Autodesk Inventor part; units mm, degrees
ref_plane "YZ Plane" through (0, 0, 0) normal (1, 0, 0) x (0, 1, 0)
ref_plane "XZ Plane" through (0, 0, 0) normal (0, 1, 0) x (-1, 0, 0)
ref_plane "XY Plane" through (0, 0, 0) normal (0, 0, 1) x (1, 0, 0)
sketch "Sketch1" plane through (0, 0, 0) normal (0, 1, 0) x (-1, 0, 0)
  line L0 (-12.7, -12.7) -> (12.7, -12.7)
  line L1 (12.7, -12.7) -> (12.7, 12.7)
  line L2 (12.7, 12.7) -> (-12.7, 12.7)
  line L3 (-12.7, 12.7) -> (-12.7, -12.7)
  line L4 (-12.7, -12.7) -> (12.7, 12.7) construction
  line L5 (12.7, -12.7) -> (-12.7, 12.7) construction
  line L6 (9.525, 9.525) -> (9.525, -9.525)
  line L7 (9.525, -9.525) -> (-9.525, -9.525)
  line L8 (-9.525, -9.525) -> (-9.525, 9.525)
  line L9 (-9.525, 9.525) -> (9.525, 9.525)
  point P0 (0, 0)
  dimension "d0" = 25.4
  dimension "d1" = 25.4
  dimension "d2" = 3.175
extrude "Extrusion1" add sketch "Sketch1" along normal blind 514.35
sketch "Sketch2" plane through (12.7, 0, 12.7) normal (1, 0, 0) x (0, 0, -1)
  line L0 (25.4, 514.35) -> (0, 514.35)
  line L1 (0, 514.35) -> (25.4, 488.95)
  line L2 (25.4, 0) -> (25.4, 514.35)
  circle A0 centre (12.7, 482.6) radius 3.2512
  line L3 (0, 514.35) -> (25.4, 514.35)
  circle A1 centre (12.7, 463.55) radius 3.2512
  circle A2 centre (12.7, 501.65) radius 3.2512
  point P0 (12.7, 0)
  point P1 (12.7, 514.35)
  point P2 (12.7, 514.35)
  point P3 (14.9989, 499.3511)
  point P4 (10.4011, 503.9489)
  dimension "d5" = 25.4
  dimension "d6" = 6.5024
  dimension "d7" = 31.75
  dimension "d8" = 19.05
extrude "Extrusion2" cut sketch "Sketch2" against normal blind 522.224
sketch "Sketch3" plane through (0, 0, 0) normal (0, -1, 0) x (1, 0, 0)
  line L0 (-12.7, -12.7) -> (-12.7, 12.7)
  line L1 (12.7, -12.7) -> (-12.7, -12.7)
  line L2 (12.7, 12.7) -> (12.7, -12.7)
  line L3 (-12.7, 12.7) -> (12.7, 12.7)
  line L4 (-9.525, 9.525) -> (-9.525, -9.525)
  line L5 (9.525, 9.525) -> (-9.525, 9.525)
  line L6 (9.525, -9.525) -> (9.525, 9.525)
  line L7 (-9.525, -9.525) -> (9.525, -9.525)
  point P0 (0, 0)
extrude "Extrusion3" cut sketch "Sketch3" against normal blind 4.7752
sketch "Sketch4" plane through (12.7, 4.7752, 12.7) normal (1, 0, 0) x (0, 0, -1)
  line L0 (0, 0) -> (25.4, 0)
  circle A0 centre (12.7, 58.7375) radius 2.4892
  point P0 (12.7, -4.7752)
  point P1 (12.7, 0)
  dimension "d13" = 4.9784
  dimension "d14" = 58.7375
extrude "Extrusion4" cut sketch "Sketch4" against normal blind 25.4
properties part number "STRU_007_BilletPole_SwerveOffset" material "Aluminum 6061"
Build history of the part. All positions in model axes, mm. A direction names the side the tool comes from. Round coordinates to 2 decimals unless told otherwise and drop trailing zeros. Write each loop counter-clockwise with the first axis right and the second up, starting at its lowest first coordinate (ties: lowest second). Pieces come first, ordered by that corner, then holes. Notation, with made-up numbers: M 85,-34.5 L 107,-34.5 A16 cw 107,-6.5 Z; hole C 83.25,65 d8. An arc over 180 degrees is marked long. Answer as a JSON object with one key per item and string values. Group by question number.
(1) Cut at A-A (x = 4). Give the cut face in (y, z) (3 decimals).
(2) Mould opens along Z. For faces 3 (the flat face through (12.7, 256, 0)), 4 (the flat face through (9.525, 254, 0)), 5 (the flat face through (0, 243, -12.7)), 6 (the flat face through (-9.525, 254, 0)) say: pulls with the +Z half, pulls with the -Z half, needs draft (parallel to the pull), parting line crosses it, or undercut.
(3) Which spindle directions (+Z, -Z, +X, -X, +Y, -Y) get a long thin tool onto all of the face, cutting with end or side? Do faces 1 (the flat face through (0, 245, -9.525)), 2 (the flat face through (0.18, 491.91, -9.74)). Say none if no direction does.
(4) Drill centre lines: L1, parallel to Y at x = 11.75, z = 0; L2, parallel to X at y = 413, z = -0.25 (3 decimals). Where is each one in solid material? Low to high.
(5) Cut at B-B (y = 333). Give the cut face in (x, z) (3 decimals), and give its area (3 significant figures).
Responses:
{
 "1": {"outline": "M 4.775,-12.7 L 488.95,-12.7 L 492.125,-9.525 L 4.775,-9.525 Z; M 4.775,9.525 L 511.175,9.525 L 514.35,12.7 L 4.775,12.7 Z"},
 "2": {"face 3": "needs draft", "face 4": "undercut", "face 5": "pulls with the -Z half", "face 6": "undercut"},
 "3": {"face 1": "+Y, -Y", "face 2": "-Z, +X, -X, +Y"},
 "4": {"L1": "y = 4.78 to 61.02, 66 to 460.3, 466.8 to 479.35, 485.85 to 498.4", "L2": "x = -12.7 to -9.525, 9.525 to 12.7"},
 "5": {"outline": "M -12.7,-12.7 L 12.7,-12.7 L 12.7,12.7 L -12.7,12.7 Z; hole M -9.525,-9.525 L 9.525,-9.525 L 9.525,9.525 L -9.525,9.525 Z", "area": "282 mm2"}
}
